Geometry: final body of the model. Coordinates: model frame, mm. Give positions to 0.01 mm unless a question says otherwise; leave off trailing zeros. Write each loop counter-clockwise with the first axis right and the second up, starting at its lowest first coordinate (ties: lowest second). Pieces come first, ordered by that corner, then holes. Notation, with made-up numbers: (-40, -8.75) -> (-2, -8.75) arc R20 ccw to (-2, 3.25) -> close; hole circle Ø11 at (-28.5, -21.5). An arc over 180 degrees is marked (long way). Answer in a Markdown table with one row per item. Add a question column.
Item 1: Section query A-A on x = 0. Output: boundary loops of the cut face in (y, z), plus the area to 3 significant figures.
Item 2: First-contact query: P1, Ø10, axis at x = -29.5, z = -14, coming from the -Y side; P2, Ø1.5, axis at y = -0.5, z = -22, coming from the -X side; P3, Ø3, axis at x = 24.5, y = -2.5, coming from the -Z side. Flat tips, straight axial feed; report the tip coordinate or a pass-through.
Item 3: Material intervals for probe 1 along Z at (x, y) = (0, -1.1); probe 2 along Z at (x, y) = (-5.5, -0.15); probe 3 along Z at (x, y) = (0, -3.55), sorted ascending. Write a range as from..to.
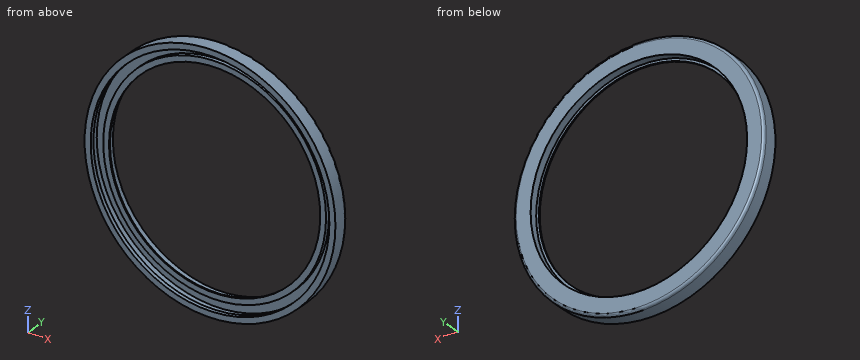
```python
from build123d import *

# Parameters (mm, degrees)
SKETCH1_R           = 47.5
BOSS_EXTRUDE1_DEPTH = 2
SKETCH2_R           = 42.25
BOSS_EXTRUDE2_DEPTH = 1.5
BOSS_EXTRUDE2_TAPER = 2
SKETCH5_R           = 10
CUT_EXTRUDE1_DEPTH  = 4
CHAMFER1_SIZE       = 1
SKETCH7_R           = 47.5
SKETCH7_R_2         = 45.7
BOSS_EXTRUDE3_DEPTH = 4
FILLET2_R           = 1
SKETCH8_R           = 41
CUT_EXTRUDE4_DEPTH  = 3
SKETCH9_R           = 40
CUT_EXTRUDE5_DEPTH  = 5
SKETCH10_R          = 45.7
SKETCH10_R_2        = 45.2
BOSS_EXTRUDE4_DEPTH = 1.5


with BuildPart() as part:
    # Sketch1 → Boss-Extrude1 (new body)
    with BuildSketch(Plane(origin=(0, 0, 0), x_dir=(1, 0, 0), z_dir=(0, 1, 0))):
        Circle(SKETCH1_R)
    extrude(amount=BOSS_EXTRUDE1_DEPTH)

    # Sketch2 → Boss-Extrude2 (add)
    with BuildSketch(Plane.XZ):
        Circle(SKETCH2_R)
    extrude(amount=BOSS_EXTRUDE2_DEPTH, taper=BOSS_EXTRUDE2_TAPER)

    # Sketch5 → Cut-Extrude1 (cut)
    with BuildSketch(Plane(origin=(0, 2, 0), x_dir=(1, 0, 0), z_dir=(0, 1, 0))):
        Circle(SKETCH5_R)
    extrude(amount=-CUT_EXTRUDE1_DEPTH, mode=Mode.SUBTRACT)

    # Chamfer1
    chamfer1_edges = [part.edges().sort_by_distance(p)[0] for p in [
        (-10, -1.5, 0),
        (-10, 2, 0),
    ]]
    chamfer(chamfer1_edges, length=CHAMFER1_SIZE)

    # Sketch7 → Boss-Extrude3 (add)
    with BuildSketch(Plane.XZ):
        Circle(SKETCH7_R)
        Circle(SKETCH7_R_2, mode=Mode.SUBTRACT)
    extrude(amount=BOSS_EXTRUDE3_DEPTH)

    # Fillet2
    fillet2_edges = [part.edges().sort_by_distance(p)[0] for p in [
        (-47.5, 2, 0),
    ]]
    fillet(fillet2_edges, radius=FILLET2_R)

    # Sketch8 → Cut-Extrude4 (cut)
    with BuildSketch(Plane(origin=(0, 2, 0), x_dir=(1, 0, 0), z_dir=(0, 1, 0))):
        Circle(SKETCH8_R)
    extrude(amount=-CUT_EXTRUDE4_DEPTH, mode=Mode.SUBTRACT)

    # Sketch9 → Cut-Extrude5 (cut)
    with BuildSketch(Plane(origin=(0, -1, 0), x_dir=(1, 0, 0), z_dir=(0, 1, 0))):
        Circle(SKETCH9_R)
    extrude(amount=-CUT_EXTRUDE5_DEPTH, mode=Mode.SUBTRACT)

    # Sketch10 → Boss-Extrude4 (add)
    with BuildSketch(Plane.XZ.offset(4)):
        Circle(SKETCH10_R)
        Circle(SKETCH10_R_2, mode=Mode.SUBTRACT)
    extrude(amount=-BOSS_EXTRUDE4_DEPTH)


solid = part.part
```
Findings below:
| question | item | result |
|---|---|---|
| 1 | outline | (-4, -47.5) -> (1, -47.5) arc R1 ccw to (2, -46.5) -> (2, -41) -> (-1, -41) -> (-1, -40) -> (-1.5, -40) -> (-1.5, -42.2) -> (0, -42.25) -> (0, -45.7) -> (-2.5, -45.7) -> (-2.5, -45.2) -> (-4, -45.2) -> close; (-4, 45.2) -> (-2.5, 45.2) -> (-2.5, 45.7) -> (0, 45.7) -> (0, 42.25) -> (-1.5, 42.2) -> (-1.5, 40) -> (-1, 40) -> (-1, 41) -> (2, 41) -> (2, 46.5) arc R1 ccw to (1, 47.5) -> (-4, 47.5) -> close |
| 1 | area | 46.1 mm^2 |
| 2 | P1 | passes through |
| 2 | P2 | stops at x = -42.48 |
| 2 | P3 | stops at z = -41.56 |
| 3 | probe 1 | z = -47.5..-45.7, -42.21..-40, 40..42.21, 45.7..47.5 |
| 3 | probe 2 | z = -47.18..-45.37, -41.89..-40.63, 40.63..41.89, 45.37..47.18 |
| 3 | probe 3 | z = -47.5..-45.2, 45.2..47.5 |
